```python
from build123d import *

# Parameters (mm, degrees)
SKETCH_1_W           = 300
SKETCH_1_H           = 145
EXTRUDE_1_DEPTH      = 81
SHELL_1_T            = -6
SKETCH_2_R           = 2.55
CUT_EXTRUDE_1_DEPTH  = 183.705363906
SKETCH_3_R           = 4.25
CUT_EXTRUDE_2_DEPTH  = 3
SKETCH_4_OUTSIDE_W   = 370.582
SKETCH_4_OUTSIDE_H   = 151.582
SKETCH_4_OUTSIDE_W_2 = 288
SKETCH_4_OUTSIDE_H_2 = 75
CUT_EXTRUDE_3_DEPTH  = 220.959087105
SKETCH_5_R           = 1.25
CUT_EXTRUDE_4_DEPTH  = 166.326948801
SKETCH_6_R           = 1.5
CUT_EXTRUDE_5_DEPTH  = 308.83315286
SKETCH_7_R           = 1.5
CUT_EXTRUDE_6_DEPTH  = 10


with BuildPart() as part:
    # ｽｹｯﾁ1 → ﾎﾞｽ - 押し出し1 (new body)
    with BuildSketch(Plane(origin=(0, 0, 0), x_dir=(1, 0, 0), z_dir=(0, 1, 0))):
        Rectangle(SKETCH_1_W, SKETCH_1_H)
    extrude(amount=EXTRUDE_1_DEPTH)

    # ｼｪﾙ1
    shell_1_openings = [part.faces().sort_by_distance(p)[0] for p in [
        (0, 81, 0),
    ]]
    offset(amount=SHELL_1_T, openings=shell_1_openings, kind=Kind.INTERSECTION)

    # ｽｹｯﾁ2 → ｶｯﾄ - 押し出し1 (cut, through all)
    with BuildSketch(Plane(origin=(0, 6, 0), x_dir=(1, 0, 0), z_dir=(0, 1, 0))):
        with Locations(Location((140, 60, 0), (0, 0, 270))):
            Circle(SKETCH_2_R)
        with Locations(Location((140, -60, 0), (0, 0, 90))):
            Circle(SKETCH_2_R)
        with Locations(Location((-22.5, -60, 0), (0, 0, 270))):
            Circle(SKETCH_2_R)
        with Locations(Location((-22.5, 60, 0), (0, 0, 90))):
            Circle(SKETCH_2_R)
    extrude(amount=-CUT_EXTRUDE_1_DEPTH, mode=Mode.SUBTRACT)

    # ｽｹｯﾁ3 → ｶｯﾄ - 押し出し2 (cut)
    with BuildSketch(Plane(origin=(0, 6, 0), x_dir=(1, 0, 0), z_dir=(0, 1, 0))):
        with Locations(Location((140, 60, 0), (0, 0, 270))):
            Circle(SKETCH_3_R)
        with Locations(Location((-22.5, 60, 0), (0, 0, 270))):
            Circle(SKETCH_3_R)
        with Locations(Location((-22.5, -60, 0), (0, 0, 270))):
            Circle(SKETCH_3_R)
        with Locations(Location((140, -60, 0), (0, 0, 270))):
            Circle(SKETCH_3_R)
    extrude(amount=-CUT_EXTRUDE_2_DEPTH, mode=Mode.SUBTRACT)

    # ｽｹｯﾁ4 outside → ｶｯﾄ - 押し出し3 (cut, through all)
    with BuildSketch(Plane(origin=(0, 0, 66.5), x_dir=(-1, 0, 0), z_dir=(0, 0, -1))):
        with Locations((0, 40.5)):
            Rectangle(SKETCH_4_OUTSIDE_W, SKETCH_4_OUTSIDE_H)
        with Locations((0, 43.5)):
            Rectangle(SKETCH_4_OUTSIDE_W_2, SKETCH_4_OUTSIDE_H_2, mode=Mode.SUBTRACT)
    extrude(amount=-CUT_EXTRUDE_3_DEPTH, mode=Mode.SUBTRACT)


with BuildPart() as cut_extrude_3_kept_piece:
    # of the separate pieces the step leaves, the one the design keeps (cut_extrude_3_pieces_kept)
    add(part.part.solids().sort_by_distance((144, 6, 72.5))[0])

    # ｽｹｯﾁ5 → ｶｯﾄ - 押し出し4 (cut, through all)
    with BuildSketch(Plane(origin=(0, 0, 66.5), x_dir=(-1, 0, 0), z_dir=(0, 0, -1))):
        with Locations((0, 5.3)):
            Circle(SKETCH_5_R)
        with Locations((-80, 5.3)):
            Circle(SKETCH_5_R)
        with Locations((80, 5.3)):
            Circle(SKETCH_5_R)
        with Locations((-144.7, 63.5)):
            Circle(SKETCH_5_R)
        with Locations((-144.7, 23.5)):
            Circle(SKETCH_5_R)
        with Locations((144.7, 23.5)):
            Circle(SKETCH_5_R)
        with Locations((144.7, 63.5)):
            Circle(SKETCH_5_R)
    extrude(amount=-CUT_EXTRUDE_4_DEPTH, mode=Mode.SUBTRACT)

    # ｽｹｯﾁ6 → ｶｯﾄ - 押し出し5 (cut, through all)
    with BuildSketch(Plane.ZY.offset(144)):
        with Locations(Location((69.5, 23.5, 0), (0, 0, 43.662612756))):
            Circle(SKETCH_6_R)
        with Locations(Location((69.5, 63.5, 0), (0, 0, 316.337387244))):
            Circle(SKETCH_6_R)
    extrude(amount=-CUT_EXTRUDE_5_DEPTH, mode=Mode.SUBTRACT)

    # ｽｹｯﾁ7 → ｶｯﾄ - 押し出し6 (cut)
    with BuildSketch(Plane.XZ.offset(-6)):
        with Locations(Location((80, 69.5, 0), (0, 0, 270))):
            Circle(SKETCH_7_R)
        with Locations(Location((0, 69.5, 0), (0, 0, 270))):
            Circle(SKETCH_7_R)
        with Locations(Location((-80, 69.5, 0), (0, 0, 270))):
            Circle(SKETCH_7_R)
    extrude(amount=-CUT_EXTRUDE_6_DEPTH, mode=Mode.SUBTRACT)


solid = cut_extrude_3_kept_piece.part
```
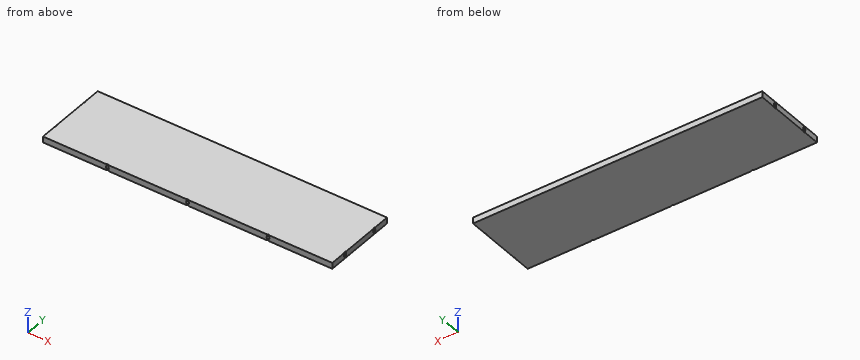
Source: CAD feature listing. Evaluate the final solid. Frame: model axes, mm. Coordinates: 2 decimals unless noted, no trailing zeros. Write each loop counter-clockwise with the first axis right and the second up, starting at its lowest first coordinate (ties: lowest second). Pieces come first, ordered by that corner, then holes. Notation, with made-up numbers: (82, 40.5) -> (118, 40.5) arc R23 ccw to (118, 79.5) -> close; hole circle Ø11 at (29, 28.5). An arc over 180 degrees is marked (long way). Return JSON: item names as keys, results as strings. Group by question number.
1) Section query A-A, the plane z = 69.5. Return loops of the section in (x, y), plus the area to 3 significant figures.
2) Section query B-B, the plane x = -74.5. Return loops of the section in (y, z), plus the area to 3 significant figures.
3) Ray query, line 1 along X through (y, z) = (13.75, 69.5); line 2 along Z through (x, y) = (-80, 11); line 3 along Y through (x, z) = (67.5, 70.5). Return the intervals inside material, ascending.
4) Contact query for flat-ended pins moving along their axis: P1, Ø2.5, axis at x = -80, z = 69.5, coming from the -Y side; P2, Ø1.8, axis at y = 63.5, z = 69.5, coming from the -X side. Output: stop coordinate, or through.
From the geometry:
{
 "1": {"outline": "(-144, 6) -> (-81.5, 6) -> (-81.5, 16) -> (-78.5, 16) -> (-78.5, 6) -> (-1.5, 6) -> (-1.5, 16) -> (1.5, 16) -> (1.5, 6) -> (78.5, 6) -> (78.5, 16) -> (81.5, 16) -> (81.5, 6) -> (144, 6) -> (144, 22) -> (-144, 22) -> close; (-144, 25) -> (144, 25) -> (144, 62) -> (-144, 62) -> close; (-144, 65) -> (144, 65) -> (144, 81) -> (-144, 81) -> close", "area": "19,800 mm²"},
 "2": {"outline": "(6, 66.5) -> (81, 66.5) -> (81, 72.5) -> (6, 72.5) -> close; hole circle Ø3 at (23.5, 69.5); hole circle Ø3 at (63.5, 69.5)", "area": "436 mm²"},
 "3": {"line 1": "-144 to -81.5, -78.5 to -1.5, 1.5 to 78.5, 81.5 to 144", "line 2": "66.5 to 68, 71 to 72.5", "line 3": "6 to 22.38, 24.62 to 62.38, 64.62 to 81"},
 "4": {"P1": "y = 16", "P2": "through"}
}
